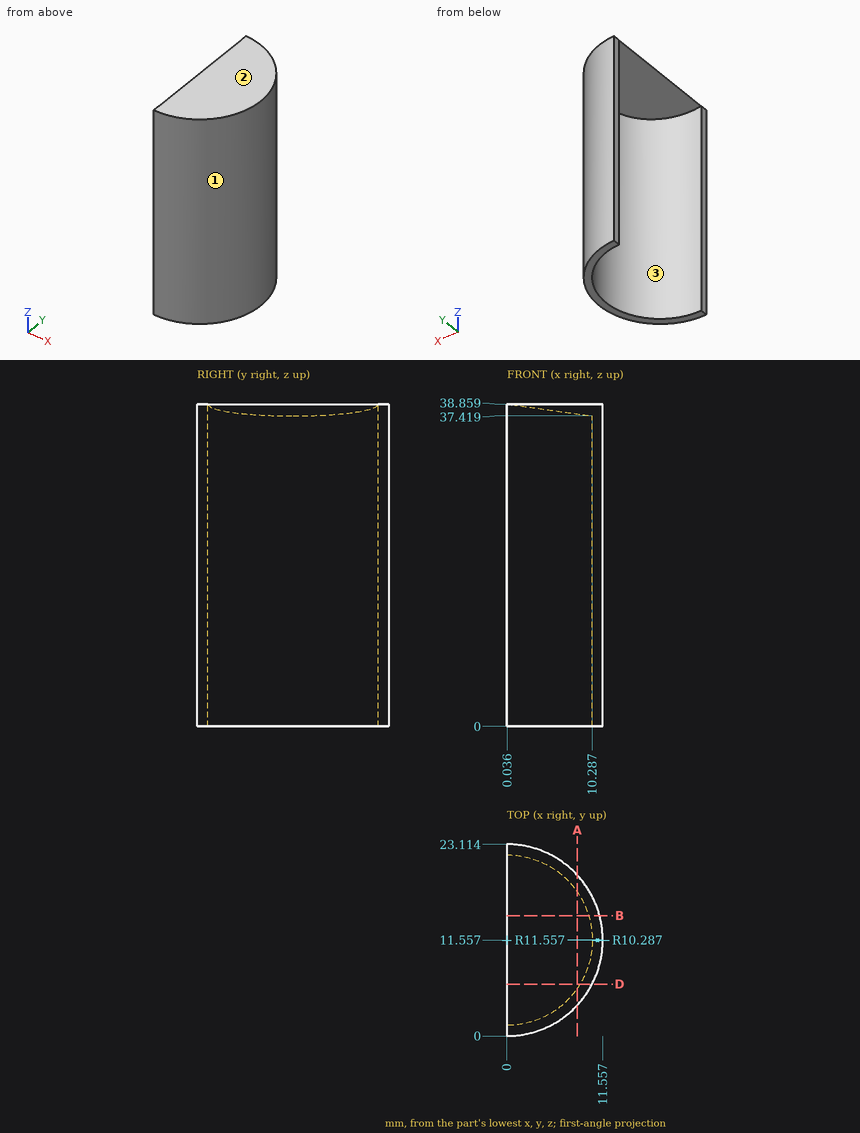
Geometry check sheet. Reference: drawing and pictorial views, mm from the part's lowest x, y, z. Give positions to 0.01 mm unless a question says otherwise; leave off trailing zeros. Order: outer loops, then holes, each group sorted by start corner. A loop starts at its lowest first (then second) coordinate and runs counter-clockwise, first axis right, second up. Notation, with made-up numbers: M 50,51 L 64,51 A26 cw 64,78 Z; hole C 33.25,-26 d11. An arc over 180 degrees is marked long. Answer in a Markdown table with one row per item. Add a question column.
Item 1: Gauge pin test, flat ends, axial feed: pin 1 (8 mm diameter, centred on y = 11, z = 29, fed in from -X); pin 2 (5 mm diameter, centred on x = 9.5, z = 8, fed in from +Y); pin 3 (1 mm diameter, centred on y = 20.5, z = 7, fed in from +X). Record the tip position at first contact, or that the pin passes through.
Item 2: Mould release check, pull along Y, two halves, no side actions. Record for the marked faces 1, 2 and 3: released by +Y, released by -Y, zero draft, split by the parting line, or undercut.
Item 3: Scan lines: probe 1 along Y at (x, z) = (0.5, 27); probe 2 along Y at (x, z) = (7.25, 5) (1 decimal); probe 3 along X at (y, z) = (18.5, 11). Record each from-to range of solid material in increasing order. Write a range as from..to.
Item 4: Section check B-B, the plane y = 14.5. Enter the section's corners in (x, z).
Item 5: Section check D-D, the plane y = 6.25. Enter the section's corners in (x, z).
Item 6: Section check A-A, the plane x = 8.5. Enter the section's corners in (y, z).
Filled sheet:
| question | item | result |
|---|---|---|
| 1 | pin 1 | stops at x = 9.22 |
| 1 | pin 2 | stops at y = 20.75 |
| 1 | pin 3 | stops at x = 7.89 |
| 2 | face 1 | split by the parting line |
| 2 | face 2 | zero draft |
| 2 | face 3 | undercut |
| 3 | probe 1 | y = 0.01..1.28, 21.83..23.1 |
| 3 | probe 2 | y = 2.6..4.3, 18.9..20.6 |
| 3 | probe 3 | x = 7.59..9.24 |
| 4 | outline | M 0.04,38.86 L 9.86,37.48 L 9.86,0 L 11.18,0 L 11.18,38.86 Z |
| 5 | outline | M 0.04,38.86 L 8.81,37.63 L 8.81,0 L 10.27,0 L 10.27,38.86 Z |
| 6 | outline | M 3.73,0 L 5.76,0 L 5.76,37.67 L 17.35,37.67 L 17.35,0 L 19.39,0 L 19.39,38.86 L 3.73,38.86 Z |
